Geometry check sheet. Reference: the model listing, model coordinates, mm. A direction names the side the tool comes from. Coordinates: 2 decimals unless noted, no trailing zeros. Loops run counter-clockwise (first coordinate to the right, second up) from the corner with the lowest first, then second, coordinate; pieces in that order, holes last. Notation, with made-up numbers: (49, 71) - (99, 71) arc R24 ccw to (99, 86) - close; hole circle Ø11 at (47.25, 2.5). An arc over 180 degrees is marked (long way). One line per item, written item: value.
from build123d import *

# Parameters (mm, degrees)
BOSS_EXTRUDE1_START = 75
SKETCH1_R           = 20
BOSS_EXTRUDE1_DEPTH = 5
SKETCH2_R           = 20
BOSS_EXTRUDE2_DEPTH = 140


with BuildPart() as part:
    # Sketch1 → Boss-Extrude1 (new body, symmetric)
    with BuildSketch(Plane.XY.offset(BOSS_EXTRUDE1_START)):
        with BuildLine():
            Line((-40, 0), (-40, 300))
            ThreePointArc((-40, 300), (0, 340), (40, 300))
            Line((40, 300), (40, 0))
            ThreePointArc((40, 0), (0, -40), (-40, 0))
        make_face()
        Circle(SKETCH1_R, mode=Mode.SUBTRACT)
    boss_extrude1 = extrude(amount=BOSS_EXTRUDE1_DEPTH, both=True)

    # Sketch2 → Boss-Extrude2 (add)
    with BuildSketch(Plane(origin=(0, 0, 70), x_dir=(-1, 0, 0), z_dir=(0, 0, -1))):
        with Locations((0, 300)):
            Circle(SKETCH2_R)
        with Locations((0, 200)):
            Circle(SKETCH2_R)
    extrude(amount=BOSS_EXTRUDE2_DEPTH)

    # Mirror2: Boss-Extrude1 across plane
    add(boss_extrude1.mirror(Plane.XY))


solid = part.part
(1) Cross-section at D-D on x = 24.5. Record the cut outline in (y, z), and give its area (3 significant figures).
Reply:
outline: (-31.62, -80) - (331.62, -80) - (331.62, -70) - (-31.62, -70) - close; (-31.62, 70) - (331.62, 70) - (331.62, 80) - (-31.62, 80) - close
area: 7,260 mm2
(2) Cross-section at B-B on y = 107. Record the cut outline in (x, z).
Reply:
outline: (-40, -80) - (40, -80) - (40, -70) - (-40, -70) - close; (-40, 70) - (40, 70) - (40, 80) - (-40, 80) - close
(3) Access from +Z, -Z, +X, -X, +Y, -Y to the whole of each face (thin tool, end or side, straight path). Record for faces 5 (the face through (-40, 148, -75)), 6 (the face through (4.336, 280.476, 0.98)).
Reply:
face 5: +Z, -Z, -X, +Y, -Y
face 6: none
(4) Release check for a two-part mould opening along Y. For faces 1 (the face through (-0.88, 339.99, 75.07)), 2 (the face through (1, 153, -70)), 3 (the face through (-40, 148, 75)), 4 (the face through (0.88, -39.99, 75.07)) record: pulls with the +Y half, pulls with the -Y half, needs draft (parallel to the pull), parting line crosses it, or undercut.
Reply:
face 1: pulls with the +Y half
face 2: undercut
face 3: needs draft
face 4: pulls with the -Y half
(5) Cross-section at C-C on z = 29. Record the cut outline in (x, y), and give its area (3 significant figures).
Reply:
outline: circle Ø40 at (0, 200); circle Ø40 at (0, 300)
area: 2,510 mm2
(6) Cross-section at A-A on x = 0. Record the cut outline in (y, z).
Reply:
outline: (-40, -80) - (-20, -80) - (-20, -70) - (-40, -70) - close; (-40, 70) - (-20, 70) - (-20, 80) - (-40, 80) - close; (20, -80) - (340, -80) - (340, -70) - (320, -70) - (320, 70) - (340, 70) - (340, 80) - (20, 80) - (20, 70) - (180, 70) - (180, -70) - (20, -70) - close; hole (220, -70) - (280, -70) - (280, 70) - (220, 70) - close
(7) Go/stop test with flat-tipped pins: pin 1 Ø5 at (y, z) = (220, -64) entering from -X; pin 2 Ø12 at (y, z) = (291, -38.5) entering from +X; pin 3 Ø1.5 at (x, z) = (-3, -13) entering from +Y. Record where each tip stops, or that it passes through.
Reply:
pin 1: x = -9.68
pin 2: x = 19.77
pin 3: y = 319.87
(8) Material ranges on probe 1 along Z at (x, y) = (24.5, 200); probe 2 along Y at (x, z) = (0, -73); probe 3 along Y at (x, z) = (12.5, -31.5), recorded low to high. Write a range as from..to.
Reply:
probe 1: -80..-70, 70..80
probe 2: -40..-20, 20..340
probe 3: 184.39..215.61, 284.39..315.61
